For this review, use the dimensioned drawing (mm, ordinates from the lowest corner) and the shaded views. A direction names the side the tool comes from. Give positions to 0.01 mm unless a question says otherwise; leave off trailing zeros. Write each loop counter-clockwise with the first axis right and the second up, starting at its lowest first coordinate (ties: lowest second). Pieces come first, ordered by that corner, then holes.
1) We need section C-C on y = 62.87. Give the boundary of the cut face in (x, z).
2) We need section B-B on y = 19.5. Give the boundary of the cut face in (x, z) (1 decimal).
3) Draft analysis for pull direction X (two halves, no side actions). For the marked faces 1, 2 and 3, state which applies: pulls with the +X half, pulls with the -X half, needs draft (parallel to the pull), parting line crosses it, or undercut.
4) For P1, Ø2.5, axis at x = 147, y = 33.5, coming from the -Z side; P2, Ø2, axis at x = 120.5, z = 38, coming from the +Y side (1 decimal), all flat-tipped, find the tip position at first contact; note any pin that passes through.
5) Wall thickness on line 1 along X through (y, z) = (63, 38); line 2 along X through (y, z) = (43, 49); line 3 along Y through (x, z) = (105, 58.35): over which ranges is each line inside the solid? List them lowest first.
6) We need section A-A on x = 105. Give the boundary of the cut face in (y, z).
7) We need section D-D on z = 4. Give the boundary of the cut face in (x, y).
8) Machinability: for the marked faces 4 and 5, which of the approach directions +Z, -Z, +X, -X, +Y, -Y give a long, thin tool a straight path to every point of the face, cutting with its end or side? Answer none if there is none.
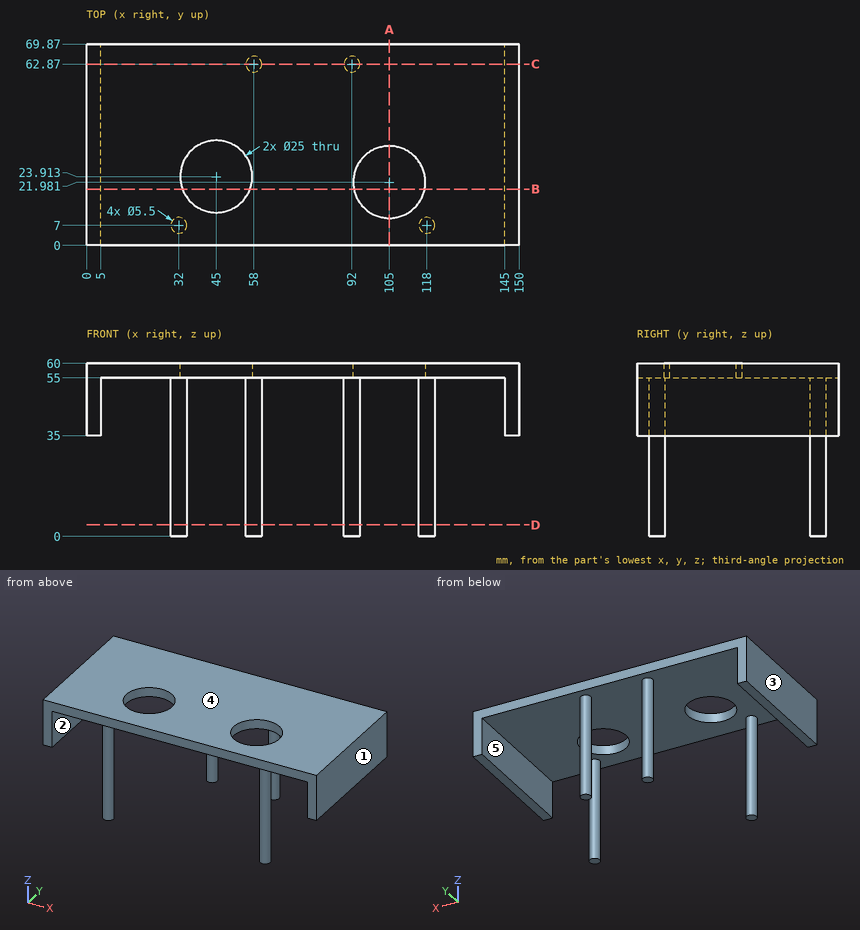
Results list:
1. outline: (0, 35) - (5, 35) - (5, 55) - (55.25, 55) - (55.25, 0) - (60.75, 0) - (60.75, 55) - (89.25, 55) - (89.25, 0) - (94.75, 0) - (94.75, 55) - (145, 55) - (145, 35) - (150, 35) - (150, 60) - (0, 60) - close
2. outline: (0, 35) - (5, 35) - (5, 55) - (33.3, 55) - (33.3, 60) - (0, 60) - close; (56.7, 55) - (92.7, 55) - (92.7, 60) - (56.7, 60) - close; (117.3, 55) - (145, 55) - (145, 35) - (150, 35) - (150, 60) - (117.3, 60) - close
3. face 1: pulls with the +X half
3. face 2: undercut
3. face 3: pulls with the -X half
4. P1: stops at z = 35
4. P2: stops at y = 9.3
5. line 1: x = 0 to 5, 55.25 to 60.75, 89.25 to 94.75, 145 to 150
5. line 2: x = 0 to 5, 145 to 150
5. line 3: y = 0 to 9.48, 34.48 to 69.87
6. outline: (0, 55) - (9.48, 55) - (9.48, 60) - (0, 60) - close; (34.48, 55) - (69.87, 55) - (69.87, 60) - (34.48, 60) - close
7. outline: circle Ø5.5 at (32, 7); circle Ø5.5 at (58, 62.87); circle Ø5.5 at (92, 62.87); circle Ø5.5 at (118, 7)
8. face 4: +Z, +X, -X, +Y, -Y
8. face 5: -Z, +Y, -Y
